The model under review builds one solid part; all positions refer to its coordinate system, in mm. Face numbers are marked on the shaded views. A direction names the side the tool comes from. Round coordinates to 2 decimals unless told otherwise and drop trailing zeros. Order: outer loops, then holes, each group sorted by start corner. A loop starts at its lowest first (then second) coordinate and runs counter-clockwise, first axis right, second up.
1) Consider section A-A (x = 4.5). Give the boundary of the cut face in (y, z).
2) Clearance check with flat-ended pins moving along their axes: P1, Ø6, axis at y = -12.5, z = -53.5, coming from the +X side; P2, Ø1.5, axis at x = 52.5, y = -3.5, coming from the +Z side; P3, Ø12, axis at y = -8.5, z = -28.5, coming from the -X side; P4, Ø2, axis at x = 55, z = -19, coming from the +Y side. State where each tip first meets the part, or that it passes through.
3) Consider section D-D (x = -31.5). Give the boundary of the cut face in (y, z).
4) Machinability: for the marked faces 4 and 5, which of the approach directions +Z, -Z, +X, -X, +Y, -Y give a long, thin tool a straight path to every point of the face, cutting with its end or side? Answer none if there is none.
5) Consider section C-C (z = -12). Give the boundary of the cut face in (x, y).
6) Consider section B-B (z = -40). Give the boundary of the cut face in (x, y).
7) To check wall thickness, follow L1, parallel to X at y = -10.75, z = 38.5; L2, parallel to Z at x = 0, y = -6; L3, parallel to Z at x = -2, y = -14.25. State the ranges of each line that lie inside material, in increasing order.
8) Mouldability with a two-part tool opening along Z and no side actions: class the marked faces 1, 2 and 3 as pulls with the +Z half, pulls with the -Z half, needs draft (parallel to the pull), parting line crosses it, or undercut.
from build123d import *

# Parameters (mm, degrees)
F0_R     = 75
F0_R_2   = 50
F1_DEPTH = 25


with BuildPart() as f1:
    # F0 (on Front) → F1 (new body)
    with BuildSketch(Plane.XZ):
        Circle(F0_R)
        Polygon((-41.721445, -53.497019), (-50.976545, -51.127983), (-53.552449, -41.928313), (-46.873254, -35.09768), (-37.618154, -37.466716), (-35.04225, -46.666385), align=None, mode=Mode.SUBTRACT)
        Polygon((8.326588, -67.329621), (0.107083, -72.198804), (-8.219505, -67.515095), (-8.326588, -57.962203), (-0.107083, -53.093021), (8.219505, -57.77673), align=None, mode=Mode.SUBTRACT)
        Polygon((53.497019, -41.721445), (51.127983, -50.976545), (41.928313, -53.552449), (35.09768, -46.873254), (37.466716, -37.618154), (46.666385, -35.04225), align=None, mode=Mode.SUBTRACT)
        Polygon((67.329621, 8.326588), (72.198804, 0.107083), (67.515095, -8.219505), (57.962203, -8.326588), (53.093021, -0.107083), (57.77673, 8.219505), align=None, mode=Mode.SUBTRACT)
        Polygon((-67.329621, -8.326588), (-72.198804, -0.107083), (-67.515095, 8.219505), (-57.962203, 8.326588), (-53.093021, 0.107083), (-57.77673, -8.219505), align=None, mode=Mode.SUBTRACT)
        Polygon((-53.497019, 41.721445), (-51.127983, 50.976545), (-41.928313, 53.552449), (-35.09768, 46.873254), (-37.466716, 37.618154), (-46.666385, 35.04225), align=None, mode=Mode.SUBTRACT)
        Circle(F0_R_2, mode=Mode.SUBTRACT)
        Polygon((-8.326588, 67.329621), (-0.107083, 72.198804), (8.219505, 67.515095), (8.326588, 57.962203), (0.107083, 53.093021), (-8.219505, 57.77673), align=None, mode=Mode.SUBTRACT)
        Polygon((41.721445, 53.497019), (50.976545, 51.127983), (53.552449, 41.928313), (46.873254, 35.09768), (37.618154, 37.466716), (35.04225, 46.666385), align=None, mode=Mode.SUBTRACT)
    extrude(amount=F1_DEPTH)


solid = f1.part
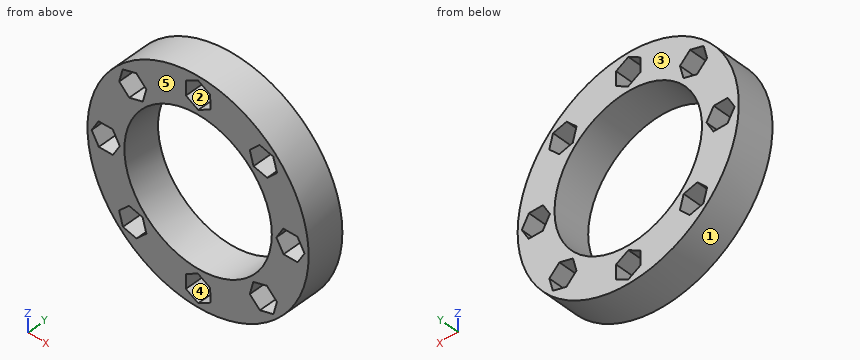
Answer below:
1. outline: (-25, -74.86) - (0, -74.86) - (0, -69.6) - (-25, -69.6) - close; (-25, -55.68) - (0, -55.68) - (0, -49.8) - (-25, -49.8) - close; (-25, 49.8) - (0, 49.8) - (0, 55.7) - (-25, 55.7) - close; (-25, 69.61) - (0, 69.61) - (0, 74.86) - (-25, 74.86) - close
2. P1: stops at x = 55.45
2. P2: stops at z = 54.29
2. P3: stops at x = -71.55
2. P4: stops at y = 0
3. outline: (-25, -68.06) - (0, -68.06) - (0, -38.83) - (-25, -38.83) - close; (-25, 38.83) - (0, 38.83) - (0, 68.06) - (-25, 68.06) - close
4. face 4: +Y, -Y
4. face 5: +Z, -Z, +X, -X, -Y
5. outline: (-74.03, -25) - (-48.54, -25) - (-48.54, 0) - (-74.03, 0) - close; (48.54, -25) - (74.03, -25) - (74.03, 0) - (48.54, 0) - close
6. outline: (-63.44, -25) - (-51.67, -25) - (-51.67, 0) - (-63.44, 0) - close; (-36.91, -25) - (-30, -25) - (-30, 0) - (-36.91, 0) - close; (30, -25) - (36.86, -25) - (36.86, 0) - (30, 0) - close; (51.74, -25) - (63.44, -25) - (63.44, 0) - (51.74, 0) - close
7. L1: x = -64.36 to -50.2, -37.24 to -31.9, 31.9 to 37.33, 50.2 to 64.36
7. L2: z = -75 to -72.14, -53.15 to -50, 50 to 53.15, 72.14 to 75
7. L3: z = -74.97 to -71.01, -54.21 to -49.96, 49.96 to 54.28, 71.08 to 74.97
8. face 1: parting line crosses it
8. face 2: undercut
8. face 3: needs draft
